from build123d import *

# Parameters (mm, degrees)
BOSS_EXTRUDE1_DEPTH = 10
SKETCH3_R           = 2
CUT_EXTRUDE1_DEPTH  = 10
SKETCH3_11_W        = 10
SKETCH3_11_H        = 26.65
SKETCH3_11_R        = 2
CUT_EXTRUDE2_DEPTH  = 7
CUT_EXTRUDE3_REACH  = 89.704
SKETCH4_W           = 9
SKETCH4_H           = 16.003442502
SKETCH4_W_2         = 18
SKETCH4_H_2         = 21
SKETCH4_H_3         = 21.24342545


with BuildPart() as part:
    # Sketch1 → Boss-Extrude1 (new body)
    with BuildSketch(Plane.XY):
        Polygon((-31, 25), (-60, 25), (-60, -29), (74, -29), (74, 36), (45, 36), (45, 46), (7, 46), (7, 41), (-31, 41), align=None)
    extrude(amount=BOSS_EXTRUDE1_DEPTH)

    # Sketch3 → Cut-Extrude1 (cut)
    with BuildSketch(Plane.XY.offset(10)):
        with BuildLine():
            ThreePointArc((-53, 22.5), (-53.585786438, 23.914213562), (-55, 24.5))
            Line((-55, 24.5), (-55, 22.5))
            Line((-55, 22.5), (-57, 22.5))
            ThreePointArc((-57, 22.5), (-55, 20.5), (-53, 22.5))
        make_face()
        with BuildLine():
            Line((-55, 22.5), (-55, 24.5))
            ThreePointArc((-55, 24.5), (-56.414213562, 23.914213562), (-57, 22.5))
            Line((-57, 22.5), (-55, 22.5))
        make_face()
        with Locations((-45, 22.5)):
            Circle(SKETCH3_R)
        with Locations((-45, -25.8)):
            Circle(SKETCH3_R)
        with Locations((-55, -25.8)):
            Circle(SKETCH3_R)
        with BuildLine():
            ThreePointArc((-17, 40.5), (-18.414213562, 39.914213562), (-19, 38.5))
            Line((-19, 38.5), (-17, 38.5))
            Line((-17, 38.5), (-17, 40.5))
        make_face()
        with BuildLine():
            Line((-17, 38.5), (-19, 38.5))
            ThreePointArc((-19, 38.5), (-17, 36.5), (-15, 38.5))
            ThreePointArc((-15, 38.5), (-15.585786438, 39.914213562), (-17, 40.5))
            Line((-17, 40.5), (-17, 38.5))
        make_face()
        with Locations((-7, 38.5)):
            Circle(SKETCH3_R)
        with Locations((-7, -9.8)):
            Circle(SKETCH3_R)
        with Locations((-17, -9.8)):
            Circle(SKETCH3_R)
        with BuildLine():
            ThreePointArc((21, 45.5), (19.585786438, 44.914213562), (19, 43.5))
            Line((19, 43.5), (21, 43.5))
            Line((21, 43.5), (21, 45.5))
        make_face()
        with BuildLine():
            Line((21, 43.5), (19, 43.5))
            ThreePointArc((19, 43.5), (21, 41.5), (23, 43.5))
            ThreePointArc((23, 43.5), (22.414213562, 44.914213562), (21, 45.5))
            Line((21, 45.5), (21, 43.5))
        make_face()
        with Locations((31, 43.5)):
            Circle(SKETCH3_R)
        with Locations((31, -4.8)):
            Circle(SKETCH3_R)
        with Locations((21, -4.8)):
            Circle(SKETCH3_R)
        with Locations((59, -14.8)):
            Circle(SKETCH3_R)
        with Locations((69, -14.8)):
            Circle(SKETCH3_R)
        with Locations((69, 33.5)):
            Circle(SKETCH3_R)
        with BuildLine():
            ThreePointArc((59, 35.5), (57.585786438, 34.914213562), (57, 33.5))
            Line((57, 33.5), (59, 33.5))
            Line((59, 33.5), (59, 35.5))
        make_face()
        with BuildLine():
            Line((59, 33.5), (57, 33.5))
            ThreePointArc((57, 33.5), (59, 31.5), (61, 33.5))
            ThreePointArc((61, 33.5), (60.414213562, 34.914213562), (59, 35.5))
            Line((59, 35.5), (59, 33.5))
        make_face()
    extrude(amount=-CUT_EXTRUDE1_DEPTH, mode=Mode.SUBTRACT)

    # Sketch3_11 → Cut-Extrude2 (cut)
    # profile 1 of 20: a face of its own
    with BuildSketch(Plane.XY.offset(10)):
        with BuildLine():
            Line((-50, 25), (-55, 25))
            Line((-55, 25), (-55, 24.5))
            ThreePointArc((-55, 24.5), (-53.585786438, 23.914213562), (-53, 22.5))
            ThreePointArc((-53, 22.5), (-55, 20.5), (-57, 22.5))
            Line((-57, 22.5), (-60, 22.5))
            Line((-60, 22.5), (-60, -1.65))
            Line((-60, -1.65), (-50, -1.65))
            Line((-50, -1.65), (-50, 25))
        make_face()
    # profile 2 of 20: a face of its own
    with BuildSketch(Plane.XY.offset(10)):
        with BuildLine():
            Line((-55, 25), (-60, 25))
            Line((-60, 25), (-60, 22.5))
            Line((-60, 22.5), (-57, 22.5))
            ThreePointArc((-57, 22.5), (-56.414213562, 23.914213562), (-55, 24.5))
            Line((-55, 24.5), (-55, 25))
        make_face()
    # profile 3 of 20: a face of its own
    with BuildSketch(Plane.XY.offset(10)):
        with Locations((-45, 11.675)):
            Rectangle(SKETCH3_11_W, SKETCH3_11_H)
        with Locations((-45, 22.5)):
            Circle(SKETCH3_11_R, mode=Mode.SUBTRACT)
    # profile 4 of 20: a face of its own
    with BuildSketch(Plane.XY.offset(10)):
        with Locations((-45, -14.975)):
            Rectangle(SKETCH3_11_W, SKETCH3_11_H)
        with Locations((-45, -25.8)):
            Circle(SKETCH3_11_R, mode=Mode.SUBTRACT)
    # profile 5 of 20: a face of its own
    with BuildSketch(Plane.XY.offset(10)):
        with Locations((-55, -14.975)):
            Rectangle(SKETCH3_11_W, SKETCH3_11_H)
        with Locations((-55, -25.8)):
            Circle(SKETCH3_11_R, mode=Mode.SUBTRACT)
    # profile 6 of 20: a face of its own
    with BuildSketch(Plane.XY.offset(10)):
        with Locations((-17, 1.025)):
            Rectangle(SKETCH3_11_W, SKETCH3_11_H)
        with Locations((-17, -9.8)):
            Circle(SKETCH3_11_R, mode=Mode.SUBTRACT)
    # profile 7 of 20: a face of its own
    with BuildSketch(Plane.XY.offset(10)):
        with Locations((-7, 1.025)):
            Rectangle(SKETCH3_11_W, SKETCH3_11_H)
        with Locations((-7, -9.8)):
            Circle(SKETCH3_11_R, mode=Mode.SUBTRACT)
    # profile 8 of 20: a face of its own
    with BuildSketch(Plane.XY.offset(10)):
        with BuildLine():
            Line((-19, 38.5), (-22, 38.5))
            Line((-22, 38.5), (-22, 14.35))
            Line((-22, 14.35), (-12, 14.35))
            Line((-12, 14.35), (-12, 41))
            Line((-12, 41), (-17, 41))
            Line((-17, 41), (-17, 40.5))
            ThreePointArc((-17, 40.5), (-15.585786438, 39.914213562), (-15, 38.5))
            ThreePointArc((-15, 38.5), (-17, 36.5), (-19, 38.5))
        make_face()
    # profile 9 of 20: a face of its own
    with BuildSketch(Plane.XY.offset(10)):
        Polygon((-2, 41), (-12, 41), (-12, 14.35), (-2, 14.35), (-2, 38.182717885), align=None)
        with Locations((-7, 38.5)):
            Circle(SKETCH3_11_R, mode=Mode.SUBTRACT)
    # profile 10 of 20: a face of its own
    with BuildSketch(Plane.XY.offset(10)):
        with BuildLine():
            Line((-17, 41), (-22, 41))
            Line((-22, 41), (-22, 38.5))
            Line((-22, 38.5), (-19, 38.5))
            ThreePointArc((-19, 38.5), (-18.414213562, 39.914213562), (-17, 40.5))
            Line((-17, 40.5), (-17, 41))
        make_face()
    # profile 11 of 20: a face of its own
    with BuildSketch(Plane.XY.offset(10)):
        with BuildLine():
            Line((19, 43.5), (16, 43.5))
            Line((16, 43.5), (16, 19.35))
            Line((16, 19.35), (26, 19.35))
            Line((26, 19.35), (26, 46))
            Line((26, 46), (21, 46))
            Line((21, 46), (21, 45.5))
            ThreePointArc((21, 45.5), (22.414213562, 44.914213562), (23, 43.5))
            ThreePointArc((23, 43.5), (21, 41.5), (19, 43.5))
        make_face()
    # profile 12 of 20: a face of its own
    with BuildSketch(Plane.XY.offset(10)):
        with Locations((31, 32.675)):
            Rectangle(SKETCH3_11_W, SKETCH3_11_H)
        with Locations((31, 43.5)):
            Circle(SKETCH3_11_R, mode=Mode.SUBTRACT)
    # profile 13 of 20: a face of its own
    with BuildSketch(Plane.XY.offset(10)):
        with BuildLine():
            Line((21, 46), (16, 46))
            Line((16, 46), (16, 43.5))
            Line((16, 43.5), (19, 43.5))
            ThreePointArc((19, 43.5), (19.585786438, 44.914213562), (21, 45.5))
            Line((21, 45.5), (21, 46))
        make_face()
    # profile 14 of 20: a face of its own
    with BuildSketch(Plane.XY.offset(10)):
        with Locations((21, 6.025)):
            Rectangle(SKETCH3_11_W, SKETCH3_11_H)
        with Locations((21, -4.8)):
            Circle(SKETCH3_11_R, mode=Mode.SUBTRACT)
    # profile 15 of 20: a face of its own
    with BuildSketch(Plane.XY.offset(10)):
        with Locations((31, 6.025)):
            Rectangle(SKETCH3_11_W, SKETCH3_11_H)
        with Locations((31, -4.8)):
            Circle(SKETCH3_11_R, mode=Mode.SUBTRACT)
    # profile 16 of 20: a face of its own
    with BuildSketch(Plane.XY.offset(10)):
        with BuildLine():
            Line((57, 33.5), (54, 33.5))
            Line((54, 33.5), (54, 9.35))
            Line((54, 9.35), (64, 9.35))
            Line((64, 9.35), (64, 36))
            Line((64, 36), (59, 36))
            Line((59, 36), (59, 35.5))
            ThreePointArc((59, 35.5), (60.414213562, 34.914213562), (61, 33.5))
            ThreePointArc((61, 33.5), (59, 31.5), (57, 33.5))
        make_face()
    # profile 17 of 20: a face of its own
    with BuildSketch(Plane.XY.offset(10)):
        with Locations((69, 22.675)):
            Rectangle(SKETCH3_11_W, SKETCH3_11_H)
        with Locations((69, 33.5)):
            Circle(SKETCH3_11_R, mode=Mode.SUBTRACT)
    # profile 18 of 20: a face of its own
    with BuildSketch(Plane.XY.offset(10)):
        with BuildLine():
            Line((59, 36), (54, 36))
            Line((54, 36), (54, 33.5))
            Line((54, 33.5), (57, 33.5))
            ThreePointArc((57, 33.5), (57.585786438, 34.914213562), (59, 35.5))
            Line((59, 35.5), (59, 36))
        make_face()
    # profile 19 of 20: a face of its own
    with BuildSketch(Plane.XY.offset(10)):
        with Locations((59, -3.975)):
            Rectangle(SKETCH3_11_W, SKETCH3_11_H)
        with Locations((59, -14.8)):
            Circle(SKETCH3_11_R, mode=Mode.SUBTRACT)
    # profile 20 of 20: a face of its own
    with BuildSketch(Plane.XY.offset(10)):
        with Locations((69, -3.975)):
            Rectangle(SKETCH3_11_W, SKETCH3_11_H)
        with Locations((69, -14.8)):
            Circle(SKETCH3_11_R, mode=Mode.SUBTRACT)
    extrude(amount=-CUT_EXTRUDE2_DEPTH, mode=Mode.SUBTRACT)


with BuildPart() as cut_extrude2_kept_piece:
    # of the separate pieces the step leaves, the one the design keeps (cut_extrude2_pieces_kept)
    add(part.part.solids().sort_by_distance((45, 36, 0))[0])

    # Sketch4 → Cut-Extrude3 (cut, up to next)
    with BuildSketch(Plane.XY.offset(10), mode=Mode.PRIVATE) as cut_extrude3_sk1:
        with Locations((-26.5, 33.001721251)):
            Rectangle(SKETCH4_W, SKETCH4_H)
    cut_extrude3_tool1 = extrude(cut_extrude3_sk1.sketch, amount=-CUT_EXTRUDE3_REACH, mode=Mode.PRIVATE) & cut_extrude2_kept_piece.part
    # Sketch4 → Cut-Extrude3 (cut, up to next)
    with BuildSketch(Plane.XY.offset(10), mode=Mode.PRIVATE) as cut_extrude3_sk2:
        with Locations((7, 35.5)):
            Rectangle(SKETCH4_W_2, SKETCH4_H_2)
    cut_extrude3_tool2 = extrude(cut_extrude3_sk2.sketch, amount=-CUT_EXTRUDE3_REACH, mode=Mode.PRIVATE) & cut_extrude2_kept_piece.part
    # Sketch4 → Cut-Extrude3 (cut, up to next)
    with BuildSketch(Plane.XY.offset(10), mode=Mode.PRIVATE) as cut_extrude3_sk3:
        with Locations((45, 35.621712725)):
            Rectangle(SKETCH4_W_2, SKETCH4_H_3)
    cut_extrude3_tool3 = extrude(cut_extrude3_sk3.sketch, amount=-CUT_EXTRUDE3_REACH, mode=Mode.PRIVATE) & cut_extrude2_kept_piece.part
    add(cut_extrude3_tool1.solids().sort_by_distance((-26.5, 33.001721, 10))[0], mode=Mode.SUBTRACT)
    add(cut_extrude3_tool2.solids().sort_by_distance((7, 35.5, 10))[0], mode=Mode.SUBTRACT)
    add(cut_extrude3_tool3.solids().sort_by_distance((45, 35.621713, 10))[0], mode=Mode.SUBTRACT)


solid = cut_extrude2_kept_piece.part
Read the model definition and answer for the solid it produces. Units are mm, in the model's axes. A direction names the side the tool comes from. Round coordinates to 2 decimals unless told otherwise and drop trailing zeros. Loops run counter-clockwise (first coordinate to the right, second up) from the corner with the lowest first, then second, coordinate; pieces in that order, holes last.
Q1. Section B-B on y = -9.8 is taken. Write down the section's boundary in (x, z), and give its area (3 significant figures).
Q2. Section C-C on z = 7.75 is taken. Write down the section's boundary in (x, y).
Q3. Section D-D on x = 31 is taken. Write down the section's boundary in (y, z).
Q4. Which of the six approach directions +Z, -Z, +X, -X, +Y, -Y give full straight-line access (tool end or side, diameter ignored) to faces 1 (the face through (26, 20, 3)), 2 (the face through (64, 36, 1)), 3 (the face through (-37, 25, 4)), 4 (the face through (64, 10, 3)), 5 (the face through (16, 35, 2))?
Q5. Determine the mould class of faces 6 (the face through (-12, 41, 1)), 7 (the face through (74, -4.2, 2.7)), 8 (the face through (-22, 33, 2)), 9 (the face through (-43.153, 21.734, 1.521)) for opening direction X: released by +X, released by -X, zero draft, split by the parting line, or undercut.
Q6. Each of these flat-tipped pins is pushed along its axis until it touches: pin 1 (4 mm diameter, centred on y = -0.5, z = 7, fed in from -X); pin 2 (1.5 mm diameter, centred on y = 32.5, z = 1.5, fed in from -X); pin 3 (3 mm diameter, centred on x = -44.5, z = 5.5, fed in from +Y). Where does it stop, or does it pass through?
Q7. Consider probe 1 along Y at (x, z) = (69, 1.2); probe 2 along X at (y, z) = (-5, 5.75); probe 3 along X at (y, z) = (-6, 1). Determine where each line is inside the solid, lowest interval first.
Q8. Section A-A on x = -45 is taken. Write down the section's boundary in (y, z).
Output:
1. outline: (-60, 0) - (-19, 0) - (-19, 3) - (-22, 3) - (-22, 10) - (-40, 10) - (-40, 3) - (-60, 3) - close; (-15, 0) - (-9, 0) - (-9, 3) - (-15, 3) - close; (-5, 0) - (74, 0) - (74, 3) - (54, 3) - (54, 10) - (-2, 10) - (-2, 3) - (-5, 3) - close
1. area: 896 mm2
2. outline: (-60, -29) - (74, -29) - (74, -17.3) - (54, -17.3) - (54, 25) - (36, 25) - (36, -7.3) - (16, -7.3) - (16, 25) - (-2, 25) - (-2, -12.3) - (-22, -12.3) - (-22, 25) - (-40, 25) - (-40, -28.3) - (-60, -28.3) - close
3. outline: (-29, 0) - (-6.8, 0) - (-6.8, 3) - (-7.3, 3) - (-7.3, 10) - (-29, 10) - close; (-2.8, 0) - (41.5, 0) - (41.5, 3) - (-2.8, 3) - close; (45.5, 0) - (46, 0) - (46, 3) - (45.5, 3) - close
4. face 1: +Z, +Y
4. face 2: +Z, -Z, +X, +Y
4. face 3: +Z, -Z, -X, +Y
4. face 4: +Z, +X, +Y
4. face 5: +Z, -Z, +Y
5. face 6: zero draft
5. face 7: released by +X
5. face 8: released by -X
5. face 9: undercut
6. pin 1: stops at x = -40
6. pin 2: stops at x = -22
6. pin 3: stops at y = -28.3
7. probe 1: y = -29 to -16.8, -12.8 to 31.5, 35.5 to 36
7. probe 2: x = -40 to -22, -2 to 16, 36 to 54
7. probe 3: x = -60 to 19.4, 22.6 to 29.4, 32.6 to 74
8. outline: (-29, 0) - (-27.8, 0) - (-27.8, 3) - (-28.3, 3) - (-28.3, 10) - (-29, 10) - close; (-23.8, 0) - (20.5, 0) - (20.5, 3) - (-23.8, 3) - close; (24.5, 0) - (25, 0) - (25, 3) - (24.5, 3) - close
